Part model, mm, in its own coordinate system. Face numbers are marked on the shaded views. Give positions to 0.01 mm unless a question says otherwise; leave off trailing zeros. Write each loop counter-clockwise with the first axis right and the second up, starting at its lowest first coordinate (ties: lowest second). Pieces come first, ordered by that corner, then holes. Notation, with made-up numbers: M 61.25,68.25 L 78.25,68.25 A17 ccw 78.25,77.25 Z; hole C 22,3.25 d11. An arc over 180 degrees is marked long. Use a Markdown table: item, result. Add a question column.
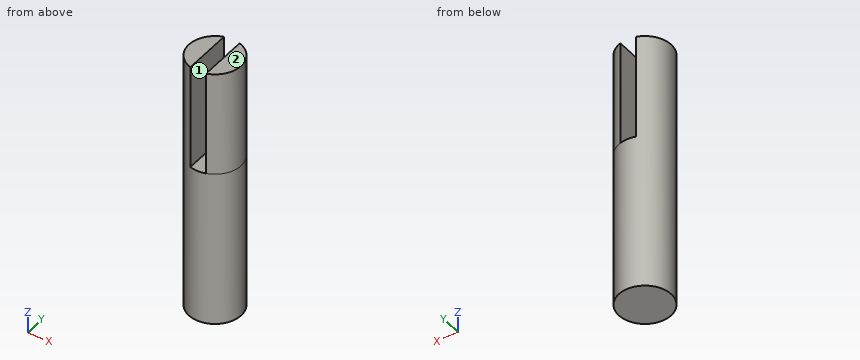
from build123d import *

# Parameters (mm, degrees)
SKETCH_R     = 2.5
PAD_DEPTH    = 15
PAD001_DEPTH = 10


with BuildPart() as part:
    # Sketch → Pad (new body)
    with BuildSketch(Plane.XY):
        Circle(SKETCH_R)
    extrude(amount=PAD_DEPTH)

    # Sketch001 (on Face3 of Pad) → Pad001 (join)
    with BuildSketch(Plane.XY.offset(15)):
        with BuildLine():
            ThreePointArc((-0.75, 2.384848), (-2.5, 0), (-0.75, -2.384848))
            Line((-0.75, -2.384848), (-0.75, 2.384848))
        make_face()
        with BuildLine():
            Line((0.75, 2.384848), (0.75, -2.384848))
            ThreePointArc((0.75, -2.384848), (2.5, 0), (0.75, 2.384848))
        make_face()
    extrude(amount=PAD001_DEPTH)


solid = part.part
1. Cut at A-A (y = 0). Write the cut outline in (x, z).
2. Cut at B-B (z = 15.75). Write the cut outline in (x, y), then the cut area to 3 significant figures.
3. Drill centre lines: probe 1 along Y at (x, z) = (-0.15, 8.25); probe 2 along Z at (x, y) = (-0.25, -2.2); probe 3 along X at (y, z) = (0.4, 22.5). Where is each one in solid material? Low to high. Write a range as [from, to].
4. Flat gauge pins, fed straight in: pin 1 (1.2 mm diameter, centred on x = 0, y = -1, fed in from +Z); pin 2 (1 mm diameter, centred on x = 0, z = 17.5, fed in from +Y). Where does each tip first touch, or does it go through?
5. Cut at C-C (x = 1.35). Write the cut outline in (y, z).
6. Mould opens along X. For the marked faces 1 and 2 say: released by +X, released by -X, zero draft, split by the parting line, or undercut.
7. Cut at D-D (y = 1.15). Write the cut outline in (x, z).
A:
| question | item | result |
|---|---|---|
| 1 | outline | M -2.5,0 L 2.5,0 L 2.5,25 L 0.75,25 L 0.75,15 L -0.75,15 L -0.75,25 L -2.5,25 Z |
| 2 | outline | M -0.75,-2.38 L -0.75,2.38 A2.5 ccw Z; M 0.75,-2.38 A2.5 ccw 0.75,2.38 Z |
| 2 | area | 12.2 mm² |
| 3 | probe 1 | y = [-2.5, 2.5] |
| 3 | probe 2 | z = [0, 15] |
| 3 | probe 3 | x = [-2.47, -0.75], [0.75, 2.47] |
| 4 | pin 1 | stops at z = 15 |
| 4 | pin 2 | passes through |
| 5 | outline | M -2.1,0 L 2.1,0 L 2.1,25 L -2.1,25 Z |
| 6 | face 1 | undercut |
| 6 | face 2 | zero draft |
| 7 | outline | M -2.22,0 L 2.22,0 L 2.22,25 L 0.75,25 L 0.75,15 L -0.75,15 L -0.75,25 L -2.22,25 Z |
